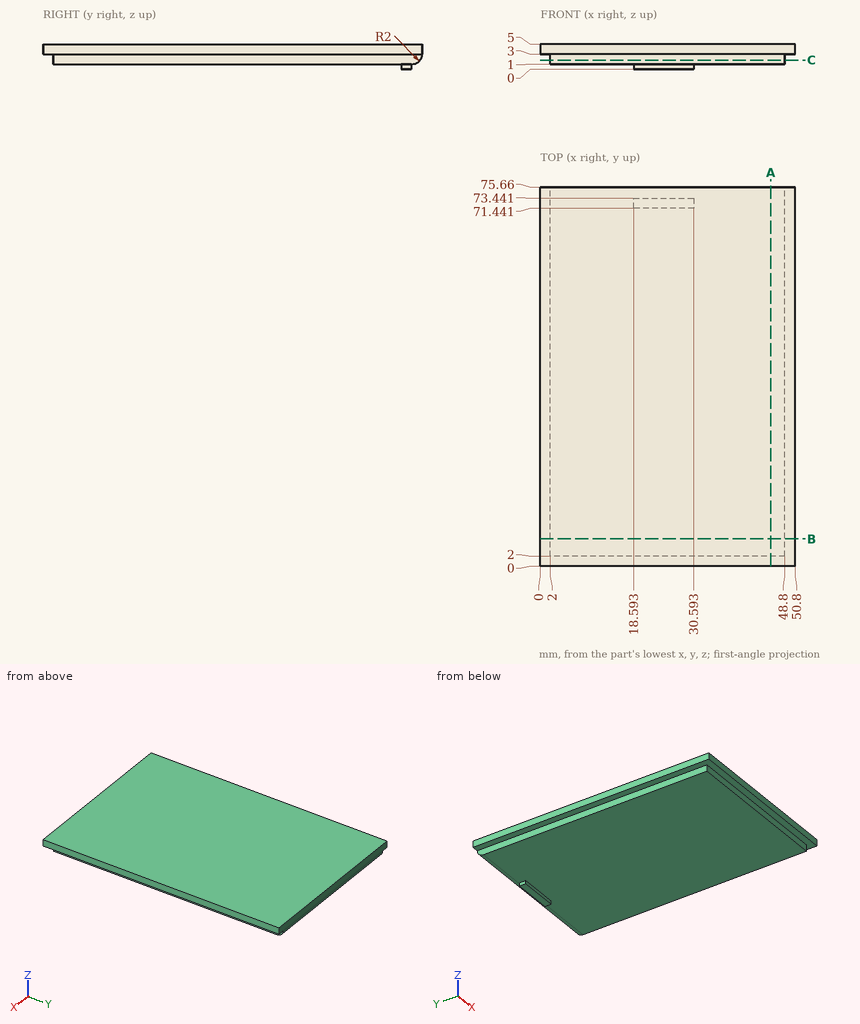
Design review of the part shown in the three views and the two pictorial views. Dimensions are in mm from the part's minimum x, y and z. Give positions to 0.01 mm unless a question says otherwise; leave off trailing zeros. Loops run counter-clockwise (first coordinate to the right, second up) from the corner with the lowest first, then second, coordinate; pieces in that order, holes last. Notation, with made-up numbers: (63.5, -40) -> (79.5, -40) arc R22 cw to (79.5, -33) -> close; hole circle Ø8 at (73.25, 32). An arc over 180 degrees is marked (long way). Put each result on its own line as item: value. Start each with the question number.
1. We need section B-B on y = 5.5. State the section outline as (x, z) points.
2. We need section C-C on z = 1.8. State the section outline as (x, y) points.
3. Wall thickness on probe 1 along Z at (x, y) = (14.5, 64); probe 2 along X at (y, z) = (57, 2.2); probe 3 along Y at (x, z) = (44, 2.5): over which ranges is each line inside the solid? List them lowest first.
4. Clearance check with flat-ended pins moving along their axes: P1, Ø2, axis at x = 34.5, y = 51.5, coming from the -Z side; P2, Ø0.8, axis at x = 27, z = 0.5, coming from the -Y side; P3, Ø0.8, axis at x = 25, z = 0.5, coming from the +Y side. State where each tip first meets the part, or that it passes through.
5. We need section A-A on x = 46. State the section outline as (y, z) points.
Determined:
1. outline: (0, 3) -> (2, 3) -> (2, 1) -> (48.8, 1) -> (48.8, 3) -> (50.8, 3) -> (50.8, 5) -> (0, 5) -> close
2. outline: (2, 2) -> (48.8, 2) -> (48.8, 75.26) -> (2, 75.26) -> close
3. probe 1: 1 to 5
3. probe 2: 2 to 48.8
3. probe 3: 2 to 75.6
4. P1: z = 1
4. P2: y = 71.44
4. P3: y = 73.44
5. outline: (0, 3) -> (2, 3) -> (2, 1) -> (73.66, 1) arc R2 ccw to (75.66, 3) -> (75.66, 5) -> (0, 5) -> close
